Input: part model. Units: mm. Frame: model coordinates. Give positions to 0.01 mm unless a question says otherwise; leave off trailing zeros. Order: outer loops, then holes, each group sorted by start corner. A loop starts at its lowest first (then second) coordinate and runs counter-clockwise, first axis right, second up. Notation, with made-up numbers: M -27,7.5 L -5,7.5 A13 cw -5,24.5 Z; hole C -19,-11.5 d1. An arc over 180 degrees is marked long. Use a Markdown table: item, result.
from build123d import *

# Parameters (mm, degrees)
SKETCH1_R             = 4.5
SKETCH1_R_2           = 3.375
BOSS_EXTRUDE1_DEPTH   = 10
CHAMFER1_SIZE         = 0.5
CHAMFER1_SIZE2        = 0.866025404
CHAMFER1_PART_2_SIZE  = 0.5
CHAMFER1_PART_2_SIZE2 = 0.866025404


with BuildPart() as part:
    # Sketch1 → Boss-Extrude1 (new body)
    with BuildSketch(Plane.XY):
        Circle(SKETCH1_R)
        Circle(SKETCH1_R_2, mode=Mode.SUBTRACT)
    extrude(amount=BOSS_EXTRUDE1_DEPTH)

    # Chamfer1
    chamfer1_edges = [part.edges().sort_by_distance(p)[0] for p in [
        (-4.5, 0, 0),
    ]]
    chamfer1_side = [part.faces().sort_by_distance(p)[0] for p in [
        (-4.372720779, 0, 0),
    ]]
    chamfer(chamfer1_edges, length=CHAMFER1_SIZE, length2=CHAMFER1_SIZE2, reference=chamfer1_side[0])

    # Chamfer1 part 2
    chamfer1_part_2_edges = [part.edges().sort_by_distance(p)[0] for p in [
        (-4.5, 0, 10),
    ]]
    chamfer1_part_2_side = [part.faces().sort_by_distance(p)[0] for p in [
        (-4.372720779, 0, 10),
    ]]
    chamfer(chamfer1_part_2_edges, length=CHAMFER1_PART_2_SIZE, length2=CHAMFER1_PART_2_SIZE2, reference=chamfer1_part_2_side[0])


solid = part.part
1) First-contact query: pin 1 Ø1.5 at (x, y) = (0, -1) entering from -Z; pin 2 Ø1 at (y, z) = (-2, 4) entering from +X; pin 3 Ø1.5 at (y, z) = (1.5, 4) entering from +X; pin 4 Ø4 at (y, z) = (2, 1) entering from -X. Flat tips, straight axial feed; report the tip coordinate or a pass-through.
Response values:
| item | result |
|---|---|
| pin 1 | passes through |
| pin 2 | stops at x = 4.24 |
| pin 3 | stops at x = 4.44 |
| pin 4 | stops at x = -4.5 |
2) Material intervals for line 1 (Y direction, x = 0, z = 3) (3 decimals); line 2 (Y direction, x = 1.5, z = 4.5); line 3 (X direction, y = -2.5, z = 8.25), sorted ascending. Write a range as from..to.
Response values:
| item | result |
|---|---|
| line 1 | y = -4.5..-3.375, 3.375..4.5 |
| line 2 | y = -4.24..-3.02, 3.02..4.24 |
| line 3 | x = -3.74..-2.27, 2.27..3.74 |
3) Cut plane A-A on y = 0. Return loops of the section in (x, z) (3 decimals), and give its area (3 significant figures).
Response values:
| item | result |
|---|---|
| outline | M -4.5,0.866 L -4,0 L -3.375,0 L -3.375,10 L -4,10 L -4.5,9.134 Z; M 3.375,0 L 4,0 L 4.5,0.866 L 4.5,9.134 L 4,10 L 3.375,10 Z |
| area | 21.6 mm² |
4) Mould query, pull axis X, two halves, no side actions, for faces 1 (the face through (-0.59, 4.46, 4.94)), 2 (the face through (-0.7, -3.3, 4.9)), 3 (the face through (-2, -3, 10)). Classes: released by +X, released by -X, zero draft, split by the parting line, or undercut.
Response values:
| item | result |
|---|---|
| face 1 | split by the parting line |
| face 2 | undercut |
| face 3 | zero draft |
5) Cut plane C-C on z = 5. Return loops of the section in (x, y) (3 decimals), and give its area (3 significant figures).
Response values:
| item | result |
|---|---|
| outline | C 0,0 d9; hole C 0,0 d6.75 |
| area | 27.8 mm² |
